```python
from build123d import *

# Parameters (mm, degrees)
F0_R     = 1.4
F1_DEPTH = 6
F2_SIZE  = 1
F3_DEPTH = 6.001
F4_DEPTH = 23


with BuildPart() as f1:
    # F0 (on Top) → F1 (new body)
    with BuildSketch(Plane.XY):
        with BuildLine():
            ThreePointArc((3.9226903411, -0.7826241038), (3.9806256647, -0.3932166296), (4, 0))
            ThreePointArc((4, 0), (3.9806256647, 0.3932166296), (3.9226903411, 0.7826241038))
            ThreePointArc((3.9226903411, 0.7826241038), (3.0310889132, 1.75), (2.639117526, 3.0058374347))
            ThreePointArc((2.639117526, 3.0058374347), (2, 3.4641016151), (1.2835728151, 3.7884615385))
            ThreePointArc((1.2835728151, 3.7884615385), (0, 3.5), (-1.2835728151, 3.7884615385))
            ThreePointArc((-1.2835728151, 3.7884615385), (-2, 3.4641016151), (-2.639117526, 3.0058374347))
            ThreePointArc((-2.639117526, 3.0058374347), (-3.0310889132, 1.75), (-3.9226903411, 0.7826241038))
            ThreePointArc((-3.9226903411, 0.7826241038), (-4, 0), (-3.9226903411, -0.7826241038))
            ThreePointArc((-3.9226903411, -0.7826241038), (-3.0310889132, -1.75), (-2.639117526, -3.0058374347))
            ThreePointArc((-2.639117526, -3.0058374347), (-2, -3.4641016151), (-1.2835728151, -3.7884615385))
            ThreePointArc((-1.2835728151, -3.7884615385), (0, -3.5), (1.2835728151, -3.7884615385))
            ThreePointArc((1.2835728151, -3.7884615385), (2, -3.4641016151), (2.639117526, -3.0058374347))
            ThreePointArc((2.639117526, -3.0058374347), (3.0310889132, -1.75), (3.9226903411, -0.7826241038))
        make_face()
        Circle(F0_R, mode=Mode.SUBTRACT)
        Circle(F0_R)
        with BuildLine():
            ThreePointArc((-1.2835728151, 3.7884615385), (0, 3.5), (1.2835728151, 3.7884615385))
            ThreePointArc((1.2835728151, 3.7884615385), (0, 4), (-1.2835728151, 3.7884615385))
        make_face()
        with BuildLine():
            ThreePointArc((2.639117526, 3.0058374347), (3.0310889132, 1.75), (3.9226903411, 0.7826241038))
            ThreePointArc((3.9226903411, 0.7826241038), (3.4641016151, 2), (2.639117526, 3.0058374347))
        make_face()
        with BuildLine():
            ThreePointArc((2.639117526, -3.0058374347), (3.4641016151, -2), (3.9226903411, -0.7826241038))
            ThreePointArc((3.9226903411, -0.7826241038), (3.0310889132, -1.75), (2.639117526, -3.0058374347))
        make_face()
        with BuildLine():
            ThreePointArc((-1.2835728151, -3.7884615385), (0, -4), (1.2835728151, -3.7884615385))
            ThreePointArc((1.2835728151, -3.7884615385), (0, -3.5), (-1.2835728151, -3.7884615385))
        make_face()
        with BuildLine():
            ThreePointArc((-3.9226903411, -0.7826241038), (-3.4641016151, -2), (-2.639117526, -3.0058374347))
            ThreePointArc((-2.639117526, -3.0058374347), (-3.0310889132, -1.75), (-3.9226903411, -0.7826241038))
        make_face()
        with BuildLine():
            ThreePointArc((-3.9226903411, 0.7826241038), (-3.0310889132, 1.75), (-2.639117526, 3.0058374347))
            ThreePointArc((-2.639117526, 3.0058374347), (-3.4641016151, 2), (-3.9226903411, 0.7826241038))
        make_face()
    extrude(amount=F1_DEPTH)

    # F2
    f2_edges = [f1.edges().sort_by_distance(p)[0] for p in [
        (2.639118, -3.005837, 6),
        (2.639118, -3.005837, 0),
    ]]
    chamfer(f2_edges, length=F2_SIZE)

    # F0 (on Top) → F3 (cut, through all)
    with BuildSketch(Plane.XY):
        with BuildLine():
            ThreePointArc((-1.2835728151, -3.7884615385), (0, -4), (1.2835728151, -3.7884615385))
            ThreePointArc((1.2835728151, -3.7884615385), (0, -3.5), (-1.2835728151, -3.7884615385))
        make_face()
        with BuildLine():
            ThreePointArc((-3.9226903411, -0.7826241038), (-3.4641016151, -2), (-2.639117526, -3.0058374347))
            ThreePointArc((-2.639117526, -3.0058374347), (-3.0310889132, -1.75), (-3.9226903411, -0.7826241038))
        make_face()
        with BuildLine():
            ThreePointArc((2.639117526, -3.0058374347), (3.4641016151, -2), (3.9226903411, -0.7826241038))
            ThreePointArc((3.9226903411, -0.7826241038), (3.0310889132, -1.75), (2.639117526, -3.0058374347))
        make_face()
        with BuildLine():
            ThreePointArc((2.639117526, 3.0058374347), (3.0310889132, 1.75), (3.9226903411, 0.7826241038))
            ThreePointArc((3.9226903411, 0.7826241038), (3.4641016151, 2), (2.639117526, 3.0058374347))
        make_face()
        with BuildLine():
            ThreePointArc((-1.2835728151, 3.7884615385), (0, 3.5), (1.2835728151, 3.7884615385))
            ThreePointArc((1.2835728151, 3.7884615385), (0, 4), (-1.2835728151, 3.7884615385))
        make_face()
        with BuildLine():
            ThreePointArc((-3.9226903411, 0.7826241038), (-3.0310889132, 1.75), (-2.639117526, 3.0058374347))
            ThreePointArc((-2.639117526, 3.0058374347), (-3.4641016151, 2), (-3.9226903411, 0.7826241038))
        make_face()
    extrude(amount=F3_DEPTH, mode=Mode.SUBTRACT)

    # F0 (on Top) → F4 (join)
    with BuildSketch(Plane.XY):
        Circle(F0_R)
    extrude(amount=-F4_DEPTH)


solid = f1.part
```
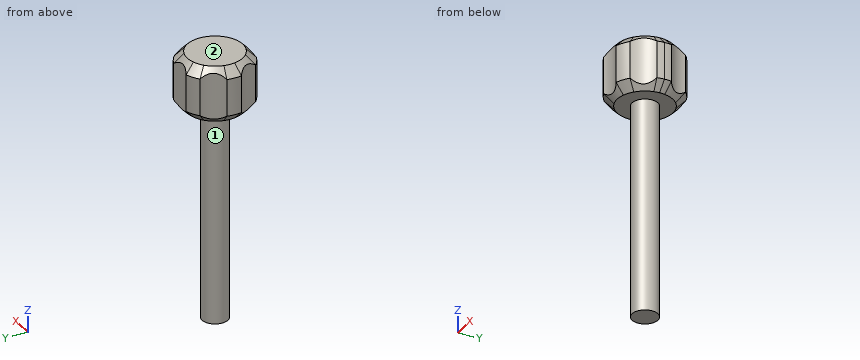
Input: part model. Units: mm. Frame: model coordinates. Face numbers are marked on the shaded views. A direction names the side the tool comes from. Give positions to 0.01 mm unless a question says otherwise; leave off trailing zeros. Order: outer loops, then holes, each group sorted by start corner. A loop starts at its lowest first (then second) coordinate and runs counter-clockwise, first axis right, second up. Notation, with made-up numbers: M 41,22.25 L 79,22.25 A16 ccw 79,28.25 Z; hole C 76.5,61 d9. An arc over 180 degrees is marked long. Return JSON: item names as keys, results as strings.
Item 1: Cut plane B-B (z = 2.75). Return loops of the section in (x, y), then the cut area to 3 significant figures.
Solutions:
{"outline": "M -3.92,-0.78 A3 cw -2.64,-3.01 A4 ccw -1.28,-3.79 A3 cw 1.28,-3.79 A4 ccw 2.64,-3.01 A3 cw 3.92,-0.78 A4 ccw 3.92,0.78 A3 cw 2.64,3.01 A4 ccw 1.28,3.79 A3 cw -1.28,3.79 A4 ccw -2.64,3.01 A3 cw -3.92,0.78 A4 ccw Z", "area": "45.1 mm^2"}
Item 2: Cut plane A-A (x = 0). Return loops of the section in (y, z).
Solutions:
{"outline": "M -3.5,0.5 L -3,0 L -1.4,0 L -1.4,-23 L 1.4,-23 L 1.4,0 L 3,0 L 3.5,0.5 L 3.5,5.5 L 3,6 L -3,6 L -3.5,5.5 Z"}
Item 3: First-contact query: P1, Ø4, axis at x = 2, z = -8.5, coming from the +Y side. Flat tip, straight axial feed; report the tip coordinate or a pass-through.
Solutions:
{"P1": "y = 1.4"}
Item 4: Access query for the marked faces 1 and 2. Directions: +Z, -Z, +X, -X, +Y, -Y. A direction counts if a zero-diameter tool reaches every point of the face in a straight line with its end or side. Return the directions, or none.
Solutions:
{"face 1": "-Z", "face 2": "+Z, +X, -X, +Y, -Y"}
Item 5: Cut plane C-C (z = -12.25). Return loops of the section in (x, y).
Solutions:
{"outline": "C 0,0 d2.8"}
Item 6: Ray query, probe 1 along Z at (x, y) = (-2, 1.25); probe 2 along Y at (x, z) = (0, 1.75); probe 3 along X at (y, z) = (-1.25, 0.25). Return the intervals inside material, ascending.
Solutions:
{"probe 1": "0 to 6", "probe 2": "-3.5 to 3.5", "probe 3": "-3 to 3"}
